```python
from build123d import *

# Parameters (mm, degrees)
F0_R         = 2.8
F1_DEPTH     = 6.5
F3_DEPTH     = 16.35
F4_T1_DEPTH  = 63.8184719387
F4_T3_DEPTH  = 45.8
F4_T5_DEPTH  = 9
F4_T7_DEPTH  = 9
F4_T10_ANGLE = 90
F4_T12_ANGLE = 120.4504110916
F4_T14_ANGLE = 90
F4_T16_ANGLE = 90
F4_T18_ANGLE = 29.7747944542
F4_T20_ANGLE = 29.7747944542
F4_T22_ANGLE = 29.7747944542
F4_T26_ANGLE = 35.5690080159
F4_T29_ANGLE = 90
F4_T33_ANGLE = 35.5690080159
F4_T36_ANGLE = 29.7747944542
F5_SIZE      = 1.56


# Not quite as in the source:
# - a fillet or chamfer that OpenCascade refuses, or shapes differently, is made with other operations: its cross-section is extruded or revolved along the edge and cut away or added


with BuildPart() as f1:
    # F0 (on Top) → F1 (new body)
    with BuildSketch(Plane.XY):
        with BuildLine():
            Line((-38.8770699501, 16.9000072956), (-38.8770699501, -28.8999927044))
            ThreePointArc((-38.8770699501, -28.8999927044), (-37.412603856, -32.4355266103), (-33.8770699501, -33.8999927044))
            Line((-33.8770699501, -33.8999927044), (29.9414019886, -33.8999927044))
            ThreePointArc((29.9414019886, -33.8999927044), (32.5106042183, -33.5643188528), (34.9073236464, -32.579832685))
            ThreePointArc((34.9073236464, -32.579832685), (50.3229300499, -5.9999927044), (34.9073236464, 20.5798472762))
            ThreePointArc((34.9073236464, 20.5798472762), (32.5106042183, 21.564333444), (29.9414019886, 21.9000072956))
            Line((29.9414019886, 21.9000072956), (-33.8770699501, 21.9000072956))
            ThreePointArc((-33.8770699501, 21.9000072956), (-37.412603856, 20.4355412015), (-38.8770699501, 16.9000072956))
        make_face()
        with Locations((-31.5170697868, -26.9999932498)):
            Circle(F0_R, mode=Mode.SUBTRACT)
        with Locations((32.2829300499, -26.9999927044)):
            Circle(F0_R, mode=Mode.SUBTRACT)
        with Locations((-31.5170697868, 15.0000071153)):
            Circle(F0_R, mode=Mode.SUBTRACT)
        with Locations((32.2829300499, 15.0000072956)):
            Circle(F0_R, mode=Mode.SUBTRACT)
    extrude(amount=F1_DEPTH)

    # F2 (on face) → F3 (join)
    with BuildSketch(Plane.XY.offset(6.5)):
        with BuildLine():
            Line((-38.8770699501, 7.9000072956), (-38.8770699501, -5.9999927044))
            Line((-38.8770699501, -5.9999927044), (-38.8770699501, -19.8999927044))
            Line((-38.8770699501, -19.8999927044), (46.9864613892, -19.8999927044))
            ThreePointArc((46.9864613892, -19.8999927044), (50.3229300499, -5.9999927044), (46.9864613892, 7.9000072956))
            Line((46.9864613892, 7.9000072956), (-38.8770699501, 7.9000072956))
        make_face()
    extrude(amount=F3_DEPTH)

    # F4: fillet of radius 0.5 on 18 edges, made by hand

    # F4_s2 → F4_t1 (cut)
    with BuildSketch(Plane.YZ.offset(-33.8770699501)):
        with BuildLine():
            ThreePointArc((21.9000072956, 0.5), (21.7535606862, 0.1464466094), (21.4000072956, 0))
            Line((21.4000072956, 0), (21.9000072956, 0))
            Line((21.9000072956, 0), (21.9000072956, 0.5))
        make_face()
        with BuildLine():
            ThreePointArc((21.9000072956, 6), (21.7535606862, 6.3535533906), (21.4000072956, 6.5))
            Line((21.4000072956, 6.5), (21.9000072956, 6.5))
            Line((21.9000072956, 6.5), (21.9000072956, 6))
        make_face()
        with BuildLine():
            ThreePointArc((-33.3999927044, 6.5), (-33.753546095, 6.3535533906), (-33.8999927044, 6))
            Line((-33.8999927044, 6), (-33.8999927044, 6.5))
            Line((-33.8999927044, 6.5), (-33.3999927044, 6.5))
        make_face()
        with BuildLine():
            ThreePointArc((-33.3999927044, 0), (-33.753546095, 0.1464466094), (-33.8999927044, 0.5))
            Line((-33.8999927044, 0.5), (-33.8999927044, 0))
            Line((-33.8999927044, 0), (-33.3999927044, 0))
        make_face()
    extrude(amount=F4_T1_DEPTH, mode=Mode.SUBTRACT)

    # F4_s4 → F4_t3 (cut)
    with BuildSketch(Plane.XZ.offset(-16.9000072956)):
        with BuildLine():
            ThreePointArc((-38.8770699501, 0.5), (-38.7306233407, 0.1464466094), (-38.3770699501, 0))
            Line((-38.3770699501, 0), (-38.8770699501, 0))
            Line((-38.8770699501, 0), (-38.8770699501, 0.5))
        make_face()
    extrude(amount=F4_T3_DEPTH, mode=Mode.SUBTRACT)

    # F4_s6 → F4_t5 (cut)
    with BuildSketch(Plane.XZ.offset(-16.9000072956)):
        with BuildLine():
            ThreePointArc((-38.8770699501, 6), (-38.7306233407, 6.3535533906), (-38.3770699501, 6.5))
            Line((-38.3770699501, 6.5), (-38.8770699501, 6.5))
            Line((-38.8770699501, 6.5), (-38.8770699501, 6))
        make_face()
    extrude(amount=F4_T5_DEPTH, mode=Mode.SUBTRACT)

    # F4_s8 → F4_t7 (cut)
    with BuildSketch(Plane.XZ.offset(19.8999927044)):
        with BuildLine():
            ThreePointArc((-38.8770699501, 6), (-38.7306233407, 6.3535533906), (-38.3770699501, 6.5))
            Line((-38.3770699501, 6.5), (-38.8770699501, 6.5))
            Line((-38.8770699501, 6.5), (-38.8770699501, 6))
        make_face()
    extrude(amount=F4_T7_DEPTH, mode=Mode.SUBTRACT)

    # F4_s9 → F4_t10 (revolve, cut)
    with BuildSketch(Plane.YZ.offset(-33.8770699501)):
        with BuildLine():
            ThreePointArc((21.9000072956, 0.5), (21.7535606862, 0.1464466094), (21.4000072956, 0))
            Line((21.4000072956, 0), (21.9000072956, 0))
            Line((21.9000072956, 0), (21.9000072956, 0.5))
        make_face()
    revolve(axis=Axis((-33.8770699501, 16.9000072956, 0), (0, 0, 1)), revolution_arc=F4_T10_ANGLE, mode=Mode.SUBTRACT)

    # F4_s11 → F4_t12 (revolve, cut)
    with BuildSketch(Plane(origin=(12.2560283734, 7.0119353437, 0), x_dir=(0, 0, 1), z_dir=(-0.8679839981, -0.4965921658, 0))):
        with BuildLine():
            ThreePointArc((0, -45.1134768811), (0.1464466094, -45.4670302717), (0.5, -45.6134768811))
            Line((0.5, -45.6134768811), (0, -45.6134768811))
            Line((0, -45.6134768811), (0, -45.1134768811))
        make_face()
    revolve(axis=Axis((19.7004300499, -5.9999927044, 0), (0, 0, 1)), revolution_arc=F4_T12_ANGLE, mode=Mode.SUBTRACT)

    # F4_s13 → F4_t14 (revolve, cut)
    with BuildSketch(Plane.YZ.offset(-33.8770699501)):
        with BuildLine():
            ThreePointArc((21.9000072956, 6), (21.7535606862, 6.3535533906), (21.4000072956, 6.5))
            Line((21.4000072956, 6.5), (21.9000072956, 6.5))
            Line((21.9000072956, 6.5), (21.9000072956, 6))
        make_face()
    revolve(axis=Axis((-33.8770699501, 16.9000072956, 6.5), (0, 0, 1)), revolution_arc=F4_T14_ANGLE, mode=Mode.SUBTRACT)

    # F4_s15 → F4_t16 (revolve, cut)
    with BuildSketch(Plane.XZ.offset(28.8999927044)):
        with BuildLine():
            ThreePointArc((-38.3770699501, 0), (-38.7306233407, 0.1464466094), (-38.8770699501, 0.5))
            Line((-38.8770699501, 0.5), (-38.8770699501, 0))
            Line((-38.8770699501, 0), (-38.3770699501, 0))
        make_face()
    revolve(axis=Axis((-33.8770699501, -28.8999927044, 0), (0, 0, 1)), revolution_arc=F4_T16_ANGLE, mode=Mode.SUBTRACT)

    # F4_s17 → F4_t18 (revolve, cut)
    with BuildSketch(Plane.YZ.offset(29.9414019886)):
        with BuildLine():
            ThreePointArc((-33.3999927044, 0), (-33.753546095, 0.1464466094), (-33.8999927044, 0.5))
            Line((-33.8999927044, 0.5), (-33.8999927044, 0))
            Line((-33.8999927044, 0), (-33.3999927044, 0))
        make_face()
    revolve(axis=Axis((29.9414019886, -23.8999927044, 0), (0, 0, 1)), revolution_arc=F4_T18_ANGLE, mode=Mode.SUBTRACT)

    # F4_s19 → F4_t20 (revolve, cut)
    with BuildSketch(Plane(origin=(17.4284307256, -9.9711770948, 0), x_dir=(0, 0, 1), z_dir=(0.8679839981, -0.4965921658, 0))):
        with BuildLine():
            ThreePointArc((0, -34.6976815693), (0.1464466094, -35.0512349599), (0.5, -35.1976815693))
            Line((0.5, -35.1976815693), (0, -35.1976815693))
            Line((0, -35.1976815693), (0, -34.6976815693))
        make_face()
    revolve(axis=Axis((29.9414019886, 11.9000072956, 0), (0, 0, 1)), revolution_arc=F4_T20_ANGLE, mode=Mode.SUBTRACT)

    # F4_s21 → F4_t22 (revolve, cut)
    with BuildSketch(Plane(origin=(17.4284307256, -9.9711770948, 0), x_dir=(0, 0, 1), z_dir=(0.8679839981, -0.4965921658, 0))):
        with BuildLine():
            ThreePointArc((6.5, -34.6976815693), (6.3535533906, -35.0512349599), (6, -35.1976815693))
            Line((6, -35.1976815693), (6.5, -35.1976815693))
            Line((6.5, -35.1976815693), (6.5, -34.6976815693))
        make_face()
    revolve(axis=Axis((29.9414019886, 11.9000072956, 6.5), (0, 0, 1)), revolution_arc=F4_T22_ANGLE, mode=Mode.SUBTRACT)


with BuildPart() as f4_tool24:
    # F4_s25 → F4_t26 (revolve)
    with BuildSketch(Plane(origin=(5.7033446243, -12.4249727464, 0), x_dir=(0, 0, 1), z_dir=(0.4171723997, -0.9088273703, 0))):
        with BuildLine():
            ThreePointArc((6.5, -45.5237586807), (6.3535533906, -45.8773120713), (6, -46.0237586807))
            Line((6, -46.0237586807), (6.5, -46.0237586807))
            Line((6.5, -46.0237586807), (6.5, -45.5237586807))
        make_face()
    revolve(axis=Axis((19.7004300499, -5.9999927044, 6.5), (0, 0, 1)), revolution_arc=F4_T26_ANGLE)

    split(bisect_by=Plane.XZ.offset(-7.9000072956), keep=Keep.BOTTOM)


with BuildPart() as f1_1:
    add(f1.part)

    # F4_t23: cut F4_tool24
    add(f4_tool24.part, mode=Mode.SUBTRACT)

    # F4_s28 → F4_t29 (revolve, cut)
    with BuildSketch(Plane.XZ.offset(28.8999927044)):
        with BuildLine():
            ThreePointArc((-38.8770699501, 6), (-38.7306233407, 6.3535533906), (-38.3770699501, 6.5))
            Line((-38.3770699501, 6.5), (-38.8770699501, 6.5))
            Line((-38.8770699501, 6.5), (-38.8770699501, 6))
        make_face()
    revolve(axis=Axis((-33.8770699501, -28.8999927044, 6.5), (0, 0, 1)), revolution_arc=F4_T29_ANGLE, mode=Mode.SUBTRACT)


with BuildPart() as f4_tool31:
    # F4_s32 → F4_t33 (revolve)
    with BuildSketch(Plane(origin=(12.2560283734, 7.0119353437, 0), x_dir=(0, 0, 1), z_dir=(-0.8679839981, -0.4965921658, 0))):
        with BuildLine():
            ThreePointArc((6.5, -45.1134768811), (6.3535533906, -45.4670302717), (6, -45.6134768811))
            Line((6, -45.6134768811), (6.5, -45.6134768811))
            Line((6.5, -45.6134768811), (6.5, -45.1134768811))
        make_face()
    revolve(axis=Axis((19.7004300499, -5.9999927044, 6.5), (0, 0, 1)), revolution_arc=F4_T33_ANGLE)

    split(bisect_by=Plane.XZ.offset(19.8999927044), keep=Keep.TOP)


with BuildPart() as f1_2:
    add(f1_1.part)

    # F4_t30: cut F4_tool31
    add(f4_tool31.part, mode=Mode.SUBTRACT)

    # F4_s35 → F4_t36 (revolve, cut)
    with BuildSketch(Plane.YZ.offset(29.9414019886)):
        with BuildLine():
            ThreePointArc((-33.3999927044, 6.5), (-33.753546095, 6.3535533906), (-33.8999927044, 6))
            Line((-33.8999927044, 6), (-33.8999927044, 6.5))
            Line((-33.8999927044, 6.5), (-33.3999927044, 6.5))
        make_face()
    revolve(axis=Axis((29.9414019886, -23.8999927044, 6.5), (0, 0, 1)), revolution_arc=F4_T36_ANGLE, mode=Mode.SUBTRACT)

    # F5
    f5_edges = [f1_2.edges().sort_by_distance(p)[0] for p in [
        (-34.31707, 15.000007, 0),
        (-34.31707, -26.999993, 0),
        (29.48293, -26.999993, 0),
        (29.48293, 15.000007, 0),
    ]]
    chamfer(f5_edges, length=F5_SIZE)


solid = f1_2.part
```
For this review, take the finished solid that the model builds, in its own axes (mm). A direction names the side the tool comes from. Round coordinates to 2 decimals unless told otherwise and drop trailing zeros. Write each loop counter-clockwise with the first axis right and the second up, starting at its lowest first coordinate (ties: lowest second). Pieces come first, ordered by that corner, then holes. Notation, with made-up numbers: (-12, -18.5) -> (35, -18.5) arc R19 cw to (35, -5.5) -> close; hole circle Ø10 at (79, 22). An arc over 180 degrees is marked (long way). One line per question, with ' | ' between items. Start each with the question number.
1) Wall thickness on line 1 along Y through (x, z) = (38, 6.75); line 2 along Z through (x, y) = (-19.5, -24); line 3 along X through (y, z) = (-0.5, 5.25): over which ranges is each line inside the solid? List them lowest first.
2) For pin 1 Ø4.5 at (x, y) = (32.28, 15) entering from +Z; pin 2 Ø1 at (x, z) = (-3.5, 18.5) entering from +Y; pin 3 Ø7 at (x, y) = (-14, 12) entering from +Z; pin 4 Ø13.5 at (x, z) = (-17, 14.5) entering from -Y, all flat-tipped, find the tip position at first contact; note any pin that passes through.
3) Mouldability with a two-part tool opening along X and no side actions: class faces 1 (the conical face through (-30, 12, 1)), 2 (the flat face through (-2, 21.9, 3)), 3 (the cylindrical face through (30.219, -25.108, 3.995)), 4 (the flat face through (-38.877, -6, 9)) as +X half, -X half, draft (parallel to the pull), parting line (faces both ways), or undercut.
4) Add section B-B (x = -23). Write out the cut boundary in (y, z).
5) Add section A-A (z = 3). Write out the cut boundary in (x, y) (1 decimal), and give its area (3 significant figures).
6) Machinability: for faces 5 (the flat face through (3, -27, 6.5)), 6 (the cylindrical face through (32.475, -33.574, 3.212)), 7 (the flat face through (3, 15, 6.5)), which of the approach directions +Z, -Z, +X, -X, +Y, -Y give a long, thin tool a straight path to every point of the face, cutting with its end or side? Answer none if there is none.
7) Add section C-C (z = 11). Write out the cut boundary in (x, y) (1 decimal).
Reported:
1) line 1: y = -19.9 to 7.9 | line 2: z = 0 to 6.5 | line 3: x = -38.88 to 49.82
2) pin 1: passes through | pin 2: stops at y = 7.9 | pin 3: stops at z = 6.5 | pin 4: stops at y = -19.9
3) face 1: undercut | face 2: draft | face 3: undercut | face 4: -X half
4) outline: (-33.9, 0.5) arc R0.5 ccw to (-33.4, 0) -> (21.4, 0) arc R0.5 ccw to (21.9, 0.5) -> (21.9, 6) arc R0.5 ccw to (21.4, 6.5) -> (7.9, 6.5) -> (7.9, 22.85) -> (-19.9, 22.85) -> (-19.9, 6.5) -> (-33.4, 6.5) arc R0.5 ccw to (-33.9, 6) -> close
5) outline: (-38.9, -28.9) arc R5 ccw to (-33.9, -33.9) -> (29.9, -33.9) arc R10 ccw to (34.9, -32.6) arc R30.6 ccw to (34.9, 20.6) arc R10 ccw to (29.9, 21.9) -> (-33.9, 21.9) arc R5 ccw to (-38.9, 16.9) -> close; hole circle Ø5.6 at (-31.5, -27); hole circle Ø5.6 at (-31.5, 15); hole circle Ø5.6 at (32.3, -27); hole circle Ø5.6 at (32.3, 15) | area: 4,590 mm²
6) face 5: +Z, +X, -X, -Y | face 6: +Z, -Z, +X, -Y | face 7: +Z, +X, -X, +Y
7) outline: (-38.9, -19.9) -> (47, -19.9) arc R30.6 ccw to (47, 7.9) -> (-38.9, 7.9) -> close
